from build123d import *

# Parameters (mm, degrees)
SKETCH1_W           = 120
SKETCH1_H           = 4
BOSS_EXTRUDE3_DEPTH = 48
SKETCH4_W           = 35
SKETCH4_H           = 4
SKETCH4_W_2         = 20
CUT_EXTRUDE2_DEPTH  = 48


with BuildPart() as part:
    # Sketch1 → Boss-Extrude3 (new body)
    with BuildSketch(Plane(origin=(0, 0, 0), x_dir=(1, 0, 0), z_dir=(0, 1, 0))):
        Rectangle(SKETCH1_W, SKETCH1_H)
    extrude(amount=BOSS_EXTRUDE3_DEPTH)

    # Sketch4 → Cut-Extrude2 (cut)
    with BuildSketch(Plane.XY.offset(2)):
        with Locations((-42.5, 46)):
            Rectangle(SKETCH4_W, SKETCH4_H)
        with Locations((0, 46)):
            Rectangle(SKETCH4_W_2, SKETCH4_H)
        with Locations((42.5, 46)):
            Rectangle(SKETCH4_W, SKETCH4_H)
        with Locations((-42.5, 2)):
            Rectangle(SKETCH4_W, SKETCH4_H)
        with Locations((0, 2)):
            Rectangle(SKETCH4_W_2, SKETCH4_H)
        with Locations((42.5, 2)):
            Rectangle(SKETCH4_W, SKETCH4_H)
    extrude(amount=-CUT_EXTRUDE2_DEPTH, mode=Mode.SUBTRACT)


solid = part.part
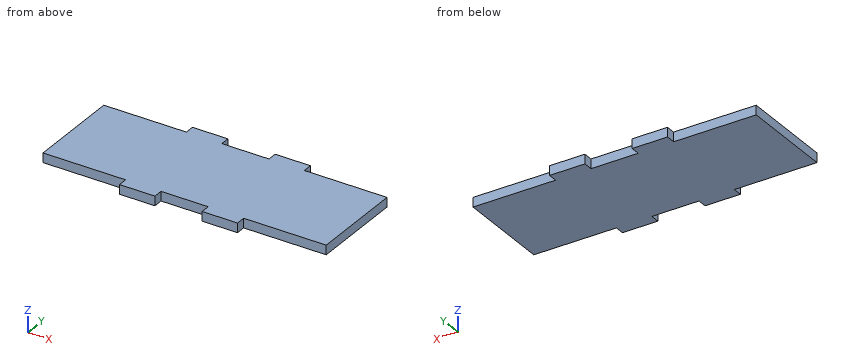
Geometry check sheet. Reference: the model listing, model coordinates, mm. Round coordinates to 2 decimals unless told otherwise and drop trailing zeros. Write each loop counter-clockwise with the first axis right and the second up, starting at its lowest first coordinate (ties: lowest second). Pieces come first, ordered by that corner, then holes.
Item 1: Material ranges on line 1 along X through (y, z) = (2, 0.3); line 2 along Y through (x, z) = (-45, 0.6), recorded low to high.
Determined:
line 1: x = -25 to -10, 10 to 25
line 2: y = 4 to 44
Item 2: Section check B-B (x = 38). Record the boundary of the cut face in (y, z), plus the area to 3 significant figures.
Determined:
outline: (4, -2) - (44, -2) - (44, 2) - (4, 2) - close
area: 160 mm2
Item 3: Go/stop test with flat-tipped pins: pin 1 Ø2 at (x, z) = (-46.5, -0.5) entering from -Y; pin 2 Ø1.2 at (y, z) = (46.5, 0) entering from -X; pin 3 Ø1.2 at (y, z) = (45.5, 0.5) entering from +X. Record where each tip stops, or that it passes through.
Determined:
pin 1: stops at y = 4
pin 2: stops at x = -25
pin 3: stops at x = 25
Item 4: Section check A-A (z = -0.9). Record the boundary of the cut face in (x, y).
Determined:
outline: (-60, 4) - (-25, 4) - (-25, 0) - (-10, 0) - (-10, 4) - (10, 4) - (10, 0) - (25, 0) - (25, 4) - (60, 4) - (60, 44) - (25, 44) - (25, 48) - (10, 48) - (10, 44) - (-10, 44) - (-10, 48) - (-25, 48) - (-25, 44) - (-60, 44) - close
